```python
from build123d import *

# Parameters (mm, degrees)
BOSS_EXTRUDE1_DEPTH = 3.175


with BuildPart() as part:
    # Sketch1 → Boss-Extrude1 (new body)
    with BuildSketch(Plane(origin=(0, 0, 0), x_dir=(1, 0, 0), z_dir=(0, 1, 0))):
        Polygon((49.775, 91.3), (19.775, 91.3), (19.775, 94.475), (0, 94.475), (0, 74.475), (3.175, 74.475), (3.175, 44.475), (0, 44.475), (0, 34), (13.275, 34), (13.275, -3.175), (56.275, -3.175), (56.275, 34), (69.55, 34), (69.55, 44.475), (66.375, 44.475), (66.375, 74.475), (69.55, 74.475), (69.55, 94.475), (49.775, 94.475), align=None)
        with BuildLine():
            add(Edge.make_bspline(
                [(24.775, 49.271255677), (24.775, 40.611001639), (39.775, 44.941128658), (54.775, 49.271255677), (39.775, 53.601382696), (24.775, 57.931509715), (24.775, 49.271255677)],
                knots=[0, 0, 0, 2.094395102, 2.094395102, 4.188790205, 4.188790205, 6.283185307, 6.283185307, 6.283185307], degree=2, weights=[1, 0.5, 1, 0.5, 1, 0.5, 1]))
        make_face(mode=Mode.SUBTRACT)
    extrude(amount=BOSS_EXTRUDE1_DEPTH)


solid = part.part
```
Geometry check sheet. Reference: the model listing, model coordinates, mm. A direction names the side the tool comes from. Round coordinates to 2 decimals unless told otherwise and drop trailing zeros. Loops run counter-clockwise (first coordinate to the right, second up) from the corner with the lowest first, then second, coordinate; pieces in that order, holes last. Notation, with made-up numbers: (35, 52.5) - (65, 52.5) arc R34 cw to (65, 88.5) - close; hole circle Ø1 at (39.25, 76.5). An arc over 180 degrees is marked (long way). Use a Markdown table: item, result.
Q1. Access from +Z, -Z, +X, -X, +Y, -Y to the whole of each face (thin tool, end or side, straight path). Record for faces 1 (the flat face through (3.175, 2, -60)), 2 (the flat face through (13.275, 2, -16)), 3 (the flat face through (66.375, 2, -59)).
Solutions:
| item | result |
|---|---|
| face 1 | -X, +Y, -Y |
| face 2 | +Z, -X, +Y, -Y |
| face 3 | +X, +Y, -Y |
Q2. Material ranges on line 1 (Z direction, x = 34.5, y = 2.15) (3 decimals); line 2 (Z direction, x = 67, y = 2.45) (3 decimals); line 3 (X direction, y = 1.6, z = -18) (3 decimals), recorded low to high.
Solutions:
| item | result |
|---|---|
| line 1 | z = -91.3 to -54.269, -44.273 to 3.175 |
| line 2 | z = -94.475 to -74.475, -44.475 to -34 |
| line 3 | x = 13.275 to 56.275 |
Q3. Draft check along X on faces 4 (the flat face through (0, 2, -39)), 5 (the flat face through (35, 2, -91.3)), 6 (the flat face through (2, 2, -44.475)), 7 (the flat face through (49.775, 2, -93)). Enter one of: released by +X, released by -X, zero draft, split by the parting line, or undercut.
Solutions:
| item | result |
|---|---|
| face 4 | released by -X |
| face 5 | undercut |
| face 6 | zero draft |
| face 7 | undercut |
Q4. Cross-section at A-A on z = -56.5. Record the cut outline in (x, y) (3 decimals).
Solutions:
| item | result |
|---|---|
| outline | (3.175, 0) - (66.375, 0) - (66.375, 3.175) - (3.175, 3.175) - close |
Q5. Cross-section at B-B on x = 8. Record the cut outline in (y, z) (3 decimals), plus the area to 3 significant figures.
Solutions:
| item | result |
|---|---|
| outline | (0, -94.475) - (3.175, -94.475) - (3.175, -34) - (0, -34) - close |
| area | 192 mm2 |
Q6. Go/stop test with flat-tipped pins: P1, Ø1.6, axis at y = 1, z = -93, coming from the -X side; P2, Ø1.6, axis at x = 32.5, y = 2.5, coming from the -Z side; P3, Ø1, axis at x = 64.5, y = 2, coming from the +Z side; P4, Ø1, axis at y = 2, z = -64.5, coming from the +X side (3 decimals). Record where each tip stops, or that it passes through.
Solutions:
| item | result |
|---|---|
| P1 | stops at x = 0 |
| P2 | stops at z = -91.3 |
| P3 | stops at z = -34 |
| P4 | stops at x = 66.375 |
